The listing builds one solid part. Answer for the finished solid, in the listing's coordinates (mm). Face numbers are marked on the shaded views. A direction names the side the tool comes from. Give positions to 0.01 mm unless a question says otherwise; leave off trailing zeros. Write each loop counter-clockwise with the first axis right and the second up, starting at its lowest first coordinate (ties: lowest second). Pieces come first, ordered by that corner, then holes. Notation, with made-up numbers: M 1.25,27 L 12.25,27 A20 ccw 12.25,49 Z; hole C 66,18 d11. An arc over 180 degrees is marked long. Return JSON: item names as keys, results as strings.
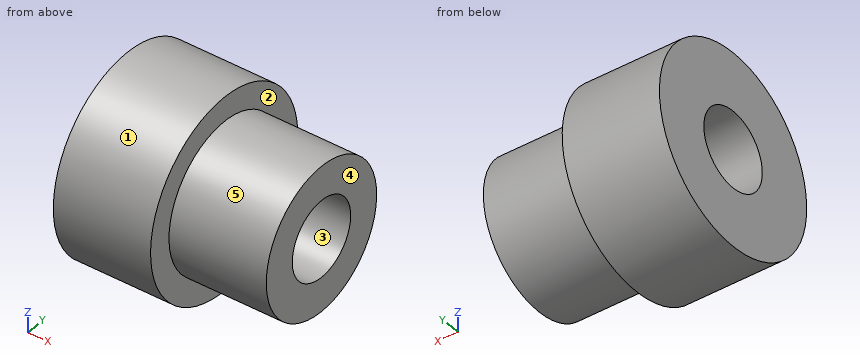
from build123d import *

# Parameters (mm, degrees)
SKETCH2_R           = 5.999999938
BOSS_EXTRUDE1_DEPTH = 8.000000002
SKETCH3_R           = 8.000000002
BOSS_EXTRUDE2_DEPTH = 8.000000002
SKETCH4_R           = 3.175
CUT_EXTRUDE1_DEPTH  = 17.000000004


with BuildPart() as part:
    # Sketch2 → Boss-Extrude1 (new body)
    with BuildSketch(Plane(origin=(0, 0, 0), x_dir=(0, 0, -1), z_dir=(1, 0, 0))):
        Circle(SKETCH2_R)
    extrude(amount=BOSS_EXTRUDE1_DEPTH)

    # Sketch3 → Boss-Extrude2 (add)
    with BuildSketch(Plane.ZY):
        Circle(SKETCH3_R)
    extrude(amount=BOSS_EXTRUDE2_DEPTH)

    # Sketch4 → Cut-Extrude1 (cut, through all)
    with BuildSketch(Plane(origin=(8.000000002, 0, 0), x_dir=(0, 0, -1), z_dir=(1, 0, 0))):
        Circle(SKETCH4_R)
    extrude(amount=-CUT_EXTRUDE1_DEPTH, mode=Mode.SUBTRACT)


solid = part.part
Item 1: A cutting plane is placed at A-A, the plane z = 0. Write down the section's boundary in (x, y) (3 decimals).
Geometry results:
{"outline": "M -8,-8 L 0,-8 L 0,-6 L 8,-6 L 8,-3.175 L -8,-3.175 Z; M -8,3.175 L 8,3.175 L 8,6 L 0,6 L 0,8 L -8,8 Z"}
Item 2: Which of the six approach directions +Z, -Z, +X, -X, +Y, -Y give full straight-line access (tool end or side, diameter ignored) to the marked faces 1 and 2?
Geometry results:
{"face 1": "+X, -X", "face 2": "+X"}
Item 3: A cutting plane is placed at D-D, the plane x = -5.25. Write down the section's boundary in (y, z) (3 decimals), plus the area to 3 significant figures.
Geometry results:
{"outline": "C 0,0 d16; hole C 0,0 d6.35", "area": "169 mm2"}
Item 4: Given pin 1 Ø4 at (x, z) = (-2.5, -5.5) entering from +Y; pin 2 Ø2 at (x, z) = (-6, -1.5) entering from +Y; pin 3 Ø2 at (x, y) = (-4.5, 6.5) entering from +Z, each flat-ended and moving along its own axis, determine where each tip first touches the part or whether it passes through.
Geometry results:
{"pin 1": "stops at y = 7.19", "pin 2": "stops at y = 7.98", "pin 3": "stops at z = 5.81"}
Item 5: Find the intervals of material crossed by line 1 (Y direction, x = 2.75, z = 0) (3 decimals); line 2 (Y direction, x = -2.75, z = 0) (3 decimals); line 3 (X direction, y = -3.75, z = -5), in increasing order.
Geometry results:
{"line 1": "y = -6 to -3.175, 3.175 to 6", "line 2": "y = -8 to -3.175, 3.175 to 8", "line 3": "x = -8 to 0"}
Item 6: A cutting plane is placed at C-C, the plane z = -4.25. Write down the section's boundary in (x, y), plus the area to 3 significant figures.
Geometry results:
{"outline": "M -8,-6.78 L 0,-6.78 L 0,-4.24 L 8,-4.24 L 8,4.24 L 0,4.24 L 0,6.78 L -8,6.78 Z", "area": "176 mm2"}
Item 7: Determine the mould class of the marked faces 3, 4 and 5 for opening direction Y: +Y half, -Y half, draft (parallel to the pull), parting line (faces both ways), or undercut.
Geometry results:
{"face 3": "undercut", "face 4": "draft", "face 5": "parting line"}
